```python
from build123d import *

# Parameters (mm, degrees)
F1_DEPTH = 25
F2_DEPTH = 24.5
F3_W     = 20
F3_H     = 10
F4_DEPTH = 1.061394367
F5_W     = 149.8626496709
F5_H     = 20
F6_DEPTH = 0.5426750459


# Not quite as in the source:
# - a feature names something its author has since deleted; it is built from what else it names


with BuildPart() as f1:
    # F0 (on Front) → F1 (new body, symmetric)
    with BuildSketch(Plane.XZ):
        Polygon((250.3392749669, 0), (-69.6607250331, 0), (-69.7979346905, 0), (-69.9352178344, -0.8798027663), (-69.8012695535, -0.9007038612), (250.3392749669, -30), align=None)
        Polygon((-69.7894617915, -0.8250317769), (-69.6638822556, -0.0320404142), (249.3347435311, -0.9683876885), (249.2535173062, -28.6408707924), align=None, mode=Mode.SUBTRACT)
        Polygon((249.3347435311, -0.9683876885), (-69.6638822556, -0.0320404142), (-69.7894617915, -0.8250317769), (249.2535173062, -28.6408707924), align=None)
    extrude(amount=F1_DEPTH, both=True)

    # F0 (on Front) → F2 (cut, symmetric)
    with BuildSketch(Plane.XZ):
        Polygon((249.3347435311, -0.9683876885), (-69.6638822556, -0.0320404142), (-69.7894617915, -0.8250317769), (249.2535173062, -28.6408707924), align=None)
    extrude(amount=F2_DEPTH, both=True, mode=Mode.SUBTRACT)

    # F3 (on face) → F4 (cut, through all)
    with BuildSketch(Plane.YZ.offset(250.3392749669)):
        with Locations((0, -15)):
            Rectangle(F3_W, F3_H)
    extrude(amount=-F4_DEPTH, mode=Mode.SUBTRACT)

    # F5 (on face) → F6 (cut, through all)
    with BuildSketch(Plane.XY):
        with Locations((29.0292073041, 0)):
            Rectangle(F5_W, F5_H)
    extrude(amount=-F6_DEPTH, mode=Mode.SUBTRACT)


solid = f1.part
```
Input: part model. Units: mm. Frame: model coordinates. A direction names the side the tool comes from. Round coordinates to 2 decimals unless told otherwise and drop trailing zeros. Write each loop counter-clockwise with the first axis right and the second up, starting at its lowest first coordinate (ties: lowest second). Pieces come first, ordered by that corner, then holes. Notation, with made-up numbers: (45, 89) -> (74, 89) arc R5 cw to (74, 94) -> close; hole circle Ø3 at (-5, 65.5). An arc over 180 degrees is marked (long way). Answer as CSV lines item,"result".
1. Section D-D (z = -7). Return the cut outline in (x, y), plus the area to 3 significant figures.
Geometry says:
outline,"(-2.7, -25) -> (250.34, -25) -> (250.34, 25) -> (-2.7, 25) -> close; hole (1.04, -24.5) -> (249.32, -24.5) -> (249.32, 24.5) -> (1.04, 24.5) -> close"
area,"486 mm^2"
2. Section A-A (y = 1). Return the cut outline in (x, z).
Geometry says:
outline,"(-69.94, -0.88) -> (-69.8, -0.9) -> (250.34, -30) -> (250.34, -20) -> (249.28, -20) -> (249.25, -28.64) -> (-69.79, -0.83) -> (-69.66, -0.03) -> (-45.9, -0.1) -> (-45.9, 0) -> (-69.8, 0) -> close; (103.96, -0.54) -> (249.33, -0.97) -> (249.31, -10) -> (250.34, -10) -> (250.34, 0) -> (103.96, 0) -> close"
3. Ray query, L1, parallel to Y at x = 183, z = -21.5; L2, parallel to Z at x = 208, y = -3.5; L3, parallel to Z at x = -4, y = 22.5. Return the intervals inside material, ascending. Write a range as [from, to].
Geometry says:
L1,"y = [-25, -24.5], [24.5, 25]"
L2,"z = [-26.15, -25.04], [-0.85, 0]"
L3,"z = [-6.88, -6.56], [-0.22, 0]"
4. Mould query, pull axis Y, two halves, no side actions, for faces 1 (the flat face through (93, -11, 0)), 2 (the flat face through (124, -25, -11)), 3 (the flat face through (123, 24.5, -11)). Classes: +Y half, -Y half, draft (parallel to the pull), parting line (faces both ways), or undercut.
Geometry says:
face 1,"draft"
face 2,"-Y half"
face 3,"undercut"
5. Section B-B (y = -18). Return the cut outline in (x, z), plus the area to 3 significant figures.
Geometry says:
outline,"(-69.94, -0.88) -> (-69.8, -0.9) -> (250.34, -30) -> (250.34, 0) -> (-69.8, 0) -> close; hole (-69.79, -0.83) -> (249.25, -28.64) -> (249.33, -0.97) -> (-69.66, -0.03) -> close"
area,"404 mm^2"
6. Reachability of faces 4 (the flat face through (123, -24.5, -11)), 5 (the flat face through (250.339, 0, -22)) from +Z, -Z, +X, -X, +Y, -Y: full face, straight path, thin tool, end or side. Return the list, or none.
Geometry says:
face 4,"none"
face 5,"+Z, -Z, +X, +Y, -Y"
7. Section C-C (x = 173). Return the cut outline in (y, z).
Geometry says:
outline,"(-25, -22.97) -> (25, -22.97) -> (25, 0) -> (-25, 0) -> close; hole (-24.5, -21.99) -> (24.5, -21.99) -> (24.5, -0.74) -> (-24.5, -0.74) -> close"
8. Contact query for flat-ended pins moving along their axis: P1, Ø5, axis at x = 77.5, y = -4.5, coming from the -Z side; P2, Ø0.8, axis at x = 249.5, y = -4, coming from the -Z side; P3, Ø0.6, axis at y = 2.5, z = -0.5, coming from the -X side. Output: stop coordinate, or through.
Geometry says:
P1,"stops at z = -14.52"
P2,"stops at z = -29.96"
P3,"stops at x = -69.92"
